Geometry: final body of the model. Coordinates: model frame, mm. Round coordinates to 2 decimals unless told otherwise and drop trailing zeros. Write each loop counter-clockwise with the first axis right and the second up, starting at its lowest first coordinate (ties: lowest second). Pieces come first, ordered by that corner, then holes. Notation, with made-up numbers: (39, -14.75) -> (77, -14.75) arc R25 ccw to (77, 17.25) -> close; hole circle Ø6 at (-20.75, 21). An arc over 180 degrees is marked (long way). Use one line per item in the form item = value. Start each with the question number.
1. Line query: L1, parallel to X at y = 2.8, z = 62.2; L2, parallel to Z at x = 0, y = 0.9; L3, parallel to Z at x = 66, y = 1.3. Output: solid intervals per line, ascending.
2. Cut plane B-B, the plane z = -2.3. Return the cut outline in (x, y).
3. Cut plane C-C, the plane x = 0. Return the cut outline in (y, z), plus the area to 3 significant figures.
4. Draft query along X for faces 1 (the face through (71.748, 2.028, -60.357)), 2 (the face through (2, 0, 30)). Return one class per face: pulls with the +X half, pulls with the -X half, needs draft (parallel to the pull), parting line crosses it, or undercut.
5. Cut plane D-D, the plane y = 1.15. State how many separate pieces and enclosed holes the cut face has, plus the area to 3 significant figures.
6. Cut plane A-A, the plane x = 66. Return the cut outline in (y, z).
7. Pin query (flat end, axial travel): pin 1 Ø1.2 at (y, z) = (1.5, 127.5) entering from -X; pin 2 Ø4 at (x, z) = (19, 22) entering from -Y; pin 3 Ø2 at (x, y) = (58, 2) entering from -Z; pin 4 Ø1.2 at (y, z) = (1.5, -44.5) entering from +X. Return the tip coordinate at first contact, or that it passes through.
Autodesk Inventor part; units mm, degrees
ref_plane "YZ Plane" through (0, 0, 0) normal (1, 0, 0) x (0, 1, 0)
ref_plane "XZ Plane" through (0, 0, 0) normal (0, 1, 0) x (-1, 0, 0)
ref_plane "XY Plane" through (0, 0, 0) normal (0, 0, 1) x (1, 0, 0)
sketch "Sketch1" plane through (0, 0, 0) normal (0, 1, 0) x (-1, 0, 0)
  line L0 (-125, 125) -> (125, 125)
  line L1 (125, 125) -> (125, -125)
  line L2 (125, -125) -> (-125, -125)
  line L3 (-125, -125) -> (-125, 125)
  line L4 (-125, 125) -> (125, -125) construction
  line L5 (125, 125) -> (-125, -125) construction
  line L6 (125, -125) -> (75, -125)
  line L7 (75, -125) -> (75, -129)
  line L8 (75, -129) -> (125, -129)
  line L9 (125, -129) -> (125, -125)
  line L10 (125, -125) -> (129, -125)
  line L11 (129, -125) -> (129, -75)
  line L12 (129, -75) -> (125, -75)
  line L13 (125, -75) -> (125, -125)
  line L14 (-125, -125) -> (-129, -125)
  line L15 (-129, -125) -> (-129, -75)
  line L16 (-129, -75) -> (-125, -75)
  line L17 (-125, -75) -> (-125, -125)
  line L18 (125, 125) -> (75, 125)
  line L19 (75, 125) -> (75, 129)
  line L20 (75, 129) -> (125, 129)
  line L21 (125, 129) -> (125, 125)
  line L22 (75, -129) -> (75, -125)
  line L23 (75, -125) -> (25, -125)
  line L24 (25, -125) -> (25, -129)
  line L25 (25, -129) -> (75, -129)
  line L26 (25, -129) -> (25, -125)
  line L27 (25, -125) -> (-25, -125)
  line L28 (-25, -125) -> (-25, -129)
  line L29 (-25, -129) -> (25, -129)
  line L30 (-25, -129) -> (-25, -125)
  line L31 (-25, -125) -> (-75, -125)
  line L32 (-75, -125) -> (-75, -129)
  line L33 (-75, -129) -> (-25, -129)
  line L34 (-75, -129) -> (-75, -125)
  line L35 (-75, -125) -> (-125, -125)
  line L36 (-125, -125) -> (-125, -129)
  line L37 (-125, -129) -> (-75, -129)
  line L38 (125, -75) -> (129, -75)
  line L39 (125, -25) -> (125, -75)
  line L40 (129, -25) -> (125, -25)
  line L41 (129, -75) -> (129, -25)
  line L42 (125, -25) -> (129, -25)
  line L43 (125, 25) -> (125, -25)
  line L44 (129, 25) -> (125, 25)
  line L45 (129, -25) -> (129, 25)
  line L46 (125, 25) -> (129, 25)
  line L47 (125, 75) -> (125, 25)
  line L48 (129, 75) -> (125, 75)
  line L49 (129, 25) -> (129, 75)
  line L50 (125, 75) -> (129, 75)
  line L51 (125, 125) -> (125, 75)
  line L52 (129, 125) -> (125, 125)
  line L53 (129, 75) -> (129, 125)
  line L54 (-125, -75) -> (-129, -75)
  line L55 (-129, -75) -> (-129, -25)
  line L56 (-129, -25) -> (-125, -25)
  line L57 (-125, -25) -> (-125, -75)
  line L58 (-125, -25) -> (-129, -25)
  line L59 (-129, -25) -> (-129, 25)
  line L60 (-129, 25) -> (-125, 25)
  line L61 (-125, 25) -> (-125, -25)
  line L62 (-125, 25) -> (-129, 25)
  line L63 (-129, 25) -> (-129, 75)
  line L64 (-129, 75) -> (-125, 75)
  line L65 (-125, 75) -> (-125, 25)
  line L66 (-125, 75) -> (-129, 75)
  line L67 (-129, 75) -> (-129, 125)
  line L68 (-129, 125) -> (-125, 125)
  line L69 (-125, 125) -> (-125, 75)
  line L70 (75, 125) -> (25, 125)
  line L71 (25, 125) -> (25, 129)
  line L72 (25, 129) -> (75, 129)
  line L73 (75, 129) -> (75, 125)
  line L74 (25, 125) -> (-25, 125)
  line L75 (-25, 125) -> (-25, 129)
  line L76 (-25, 129) -> (25, 129)
  line L77 (25, 129) -> (25, 125)
  line L78 (-25, 125) -> (-75, 125)
  line L79 (-75, 125) -> (-75, 129)
  line L80 (-75, 129) -> (-25, 129)
  line L81 (-25, 129) -> (-25, 125)
  line L82 (-75, 125) -> (-125, 125)
  line L83 (-125, 125) -> (-125, 129)
  line L84 (-125, 129) -> (-75, 129)
  line L85 (-75, 129) -> (-75, 125)
  point P0 (0, 0)
  dimension "d0" = 250
  dimension "d1" = 250
  dimension "d2" = 50
  dimension "d3" = 4
  dimension "d4" = 4
  dimension "d5" = 50
  dimension "d6" = 4
  dimension "d7" = 50
  dimension "d8" = 50
  dimension "d9" = 4
  dimension "d12" = 50
  dimension "d19" = 50
  dimension "d26" = 50
  dimension "d33" = 50
extrude "Extrusion1" add sketch "Sketch1" along normal blind 4 contours L83 L84 L79 L0 | L0 L1 L2 L3 | L3 L64 L67 L68 | L75 L76 L71 L0 | L3 L56 L59 L60 | L19 L20 L21 L0 | L3 L14 L15 L16 | L52 L53 L48 L1 | L2 L32 L37 L36 | L44 L45 L40 L1 | L2 L24 L29 L28 | L12 L11 L10 L1 | L2 L9 L8 L7
sketch "Sketch2" plane through (0, 4, 0) normal (0, 1, 0) x (1, 0, 0)
  line L0 (25, -125) -> (75, -125) construction
  circle A0 centre (0, 2.3) radius 6.5
  circle A1 centre (-66, -62.2) radius 4
  circle A2 centre (66, -62.2) radius 4
  line L1 (0, 180.6) -> (0, -180.6) construction
  line L2 (-93.2324, -124) -> (95.467, -124) construction
  line L3 (-129, -125) -> (-125, -125)
  line L4 (25, -29.4721) -> (29.2426, -25.2294)
  line L5 (44.799, -9.6731) -> (47.6274, -12.5015)
  line L6 (47.6274, -12.5015) -> (43.3848, -16.7442)
  line L7 (27.8284, -32.3005) -> (25, -29.4721)
  line L8 (34.8995, -39.3716) -> (39.1421, -35.1289)
  line L9 (54.6985, -19.5726) -> (57.5269, -22.401)
  line L10 (57.5269, -22.401) -> (53.2843, -26.6437)
  line L11 (37.7279, -42.2) -> (34.8995, -39.3716)
  line L12 (40.5563, -13.9157) -> (43.3848, -16.7442)
  line L13 (29.2426, -25.2294) -> (32.0711, -28.0579)
  line L14 (39.1421, -35.1289) -> (41.9706, -37.9574)
  line L15 (50.4558, -23.8152) -> (53.2843, -26.6437)
  line L16 (40.5563, -13.9157) -> (44.799, -9.6731)
  line L17 (29.2426, -25.2294) -> (40.5563, -13.9157) construction
  line L18 (43.3848, -16.7442) -> (32.0711, -28.0579) construction
  line L19 (50.4558, -23.8152) -> (54.6985, -19.5726)
  line L20 (53.2843, -26.6437) -> (41.9706, -37.9574) construction
  line L21 (32.0711, -28.0579) -> (27.8284, -32.3005)
  line L22 (39.1421, -35.1289) -> (50.4558, -23.8152) construction
  line L23 (41.9706, -37.9574) -> (37.7279, -42.2)
  point P0 (0, 0)
  point P1 (26.4142, -30.8863)
  dimension "d46" = 13
  dimension "d52" = 8
  dimension "d53" = 132
  dimension "d54" = 61.8
  dimension "d55" = 1
  dimension "d56" = 64.5
  dimension "d57" = 10
  dimension "d58" = 4
  dimension "d59" = 6
  dimension "d60" = 6
  dimension "d61" = 45
  dimension "d62" = 20
  dimension "d63" = 28
  dimension "d64" = 25
extrude "Extrusion2" cut sketch "Sketch2" against normal up to next
sketch "Sketch3" plane through (0, 4, 0) normal (0, 1, 0) x (1, 0, 0)
  point P0 (0, 0)
sketch "Sketch4" plane through (0, 4, 0) normal (0, 1, 0) x (1, 0, 0)
  circle A0 centre (75, 75) radius 15
  line L0 (75, 125) -> (25, 125)
  line L1 (125, 25) -> (125, 75)
  point P0 (0, 0)
  dimension "d65" = 30
  dimension "d66" = 50
  dimension "d67" = 50
extrude "Extrusion3" cut sketch "Sketch4" against normal blind 10
sketch "Sketch5" plane through (0, 4, 0) normal (0, 1, 0) x (1, 0, 0)
  line L0 (-80.4142, -24.3431) -> (-77.5858, -21.5147)
  line L1 (-77.5858, -21.5147) -> (-81.8284, -17.2721)
  line L2 (-81.8284, -17.2721) -> (-84.6569, -20.1005)
  line L3 (-84.6569, -20.1005) -> (-80.4142, -24.3431)
  line L4 (-79, -30) -> (-71.9289, -22.9289) construction
  line L5 (-83.2426, -18.6863) -> (-79, -22.9289) construction
  line L6 (-79, -22.9289) -> (-75.4645, -26.4645) construction
  line L7 (-75, -125) -> (-25, -125)
  line L8 (-125, -25) -> (-125, -75)
  point P0 (0, 0)
  dimension "d70" = 45
  dimension "d71" = 6
  dimension "d72" = 4
  dimension "d73" = 10
  dimension "d74" = 5
  dimension "d75" = 46
  dimension "d76" = 95
extrude "Extrusion4" cut sketch "Sketch5" against normal through all
properties part number "FloorPlateTop_V2" material "Wood (Oak)"
Outcome:
q1.L1 = -125 to -70, -62 to 62, 70 to 125
q1.L2 = -129 to -8.8, 4.2 to 129
q1.L3 = -125 to -87, -63 to 58.2, 66.2 to 125
q2.outline = (-129, 0) -> (-6.5, 0) -> (-6.5, 4) -> (-129, 4) -> close; (6.5, 0) -> (129, 0) -> (129, 4) -> (6.5, 4) -> close
q3.outline = (0, -129) -> (4, -129) -> (4, -8.8) -> (0, -8.8) -> close; (0, 4.2) -> (4, 4.2) -> (4, 129) -> (0, 129) -> close
q3.area = 980 mm^2
q4.face_1 = undercut
q4.face_2 = needs draft
q5.separate_pieces = 1
q5.enclosed_holes = 9
q5.area = 63,800 mm^2
q6.outline = (0, -125) -> (4, -125) -> (4, -87) -> (0, -87) -> close; (0, -63) -> (4, -63) -> (4, 58.2) -> (0, 58.2) -> close; (0, 66.2) -> (4, 66.2) -> (4, 125) -> (0, 125) -> close
q7.pin_1 = -125
q7.pin_2 = 0
q7.pin_3 = -125
q7.pin_4 = 125
